The drawing under review shows one solid part. Ordinate dimensions are in mm from its lowest x, y, z. A direction names the side the tool comes from. Coordinates: 2 decimals unless noted, no trailing zeros. Loops run counter-clockwise (first coordinate to the right, second up) from the corner with the lowest first, then second, coordinate; pieces in that order, holes last. Notation, with made-up numbers: M 34,-30 L 40,-30 A10 cw 40,-12 Z; hole C 80.25,84.25 d5. An arc over 180 degrees is marked long. Answer as a JSON object with one key per item and string values. Group by question number.
1. Machinability: for the marked faces 1, 2 and 3, which of the approach directions +Z, -Z, +X, -X, +Y, -Y give a long, thin tool a straight path to every point of the face, cutting with its end or side? Answer none if there is none.
2. Insertion check: pin 1 (6 mm diameter, centred on x = 17.5, z = 2.5, fed in from -Y); pin 2 (4.5 mm diameter, centred on y = 3.5, z = 10, fed in from +X); pin 3 (1 mm diameter, centred on y = 6, z = 2, fed in from -X); pin 4 (5 mm diameter, centred on x = 18, y = 6, fed in from +Z). Each pin has a flat end and moves straight along its axis. Give the tip position at first contact, or say it passes through.
3. Consider section B-B (z = 9.5). State the section outline as (x, y) points (1 decimal).
4. To check wall thickness, follow probe 1 along X at (y, z) = (8.5, 11.5) (1 decimal); probe 2 along Z at (x, y) = (15.25, 6); probe 3 along X at (y, z) = (6.75, 5.75) (1 decimal). State the ranges of each line that lie inside material, in increasing order.
5. Consider section C-C (x = 16.25). State the section outline as (y, z) points.
6. Consider section A-A (y = 6.5). State the section outline as (x, z) points (1 decimal).
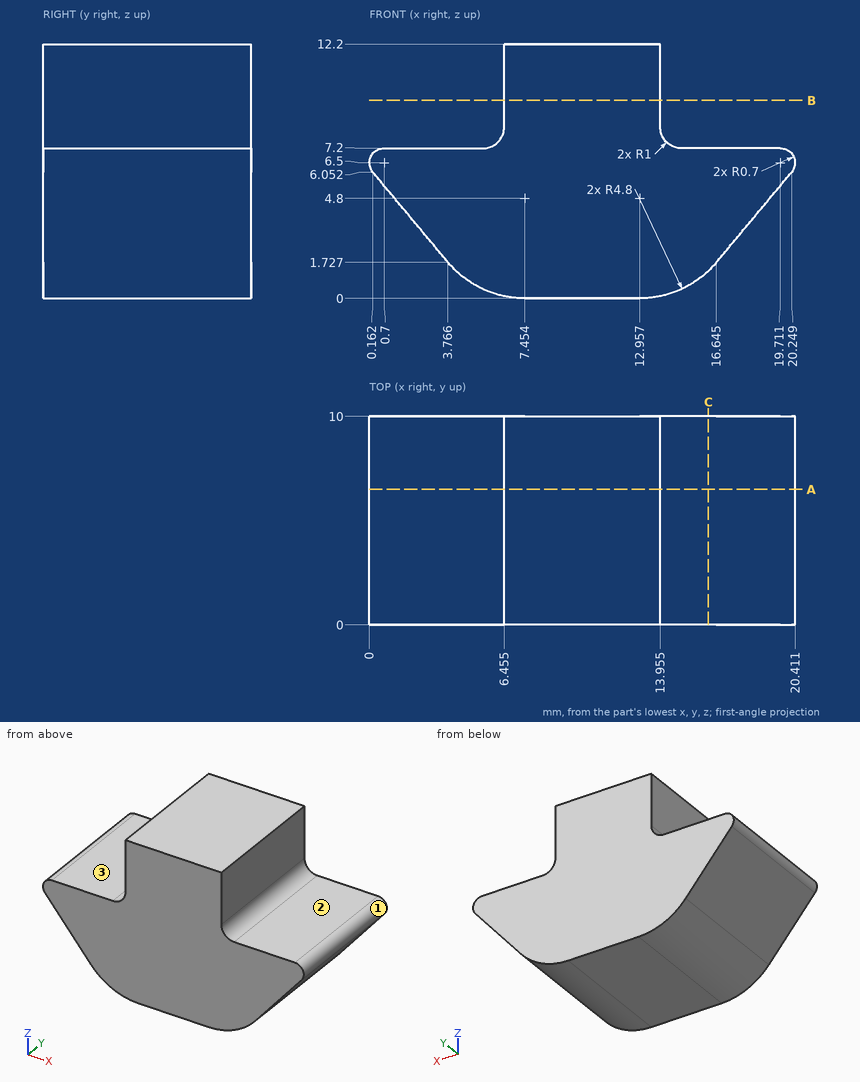
Findings below:
{
 "1": {"face 1": "+X, +Y, -Y", "face 2": "+Z, +X, +Y, -Y", "face 3": "+Z, -X, +Y, -Y"},
 "2": {"pin 1": "stops at y = 0", "pin 2": "stops at x = 14.06", "pin 3": "stops at x = 3.12", "pin 4": "stops at z = 7.2"},
 "3": {"outline": "M 6.5,0 L 14,0 L 14,10 L 6.5,10 Z"},
 "4": {"probe 1": "x = 6.5 to 14", "probe 2": "z = 0.58 to 7.2", "probe 3": "x = 0.4 to 20"},
 "5": {"outline": "M 0,1.31 L 10,1.31 L 10,7.2 L 0,7.2 Z"},
 "6": {"outline": "M 0.2,6.1 L 3.8,1.7 A4.8 ccw 7.5,0 L 13,0 A4.8 ccw 16.6,1.7 L 20.2,6.1 A0.7 ccw 19.7,7.2 L 15,7.2 A1 cw 14,8.2 L 14,12.2 L 6.5,12.2 L 6.5,8.2 A1 cw 5.5,7.2 L 0.7,7.2 A0.7 ccw Z"}
}
